Here's the drawing with two shaded views (mm, measured from the low corner). I have some questions. Give positions to 0.01 mm unless a question says otherwise; leave off trailing zeros. Loops run counter-clockwise (first coordinate to the right, second up) from the corner with the lowest first, then second, coordinate; pieces in that order, holes last. Notation, with made-up numbers: (-35.5, 48.25) -> (14.5, 48.25) arc R33 cw to (14.5, 85.25) -> close; hole circle Ø6 at (76.5, 48.5). An arc over 180 degrees is marked (long way). Answer in a Markdown table with one row per item. Add a question column.
Item 1: If we section it at B-B (x = 4): Write out the boundary of the cut face in (y, z), then the cut area to 3 significant figures.
Item 2: If we section it at A-A (z = 12.5): Write out the boundary of the cut face in (x, y).
Item 3: If I drill on line 1 (X direction, y = 25, z = 12.5); line 2 (X direction, y = 43, z = 11.75), over which ranges is the centre line in solid material (lowest first)?
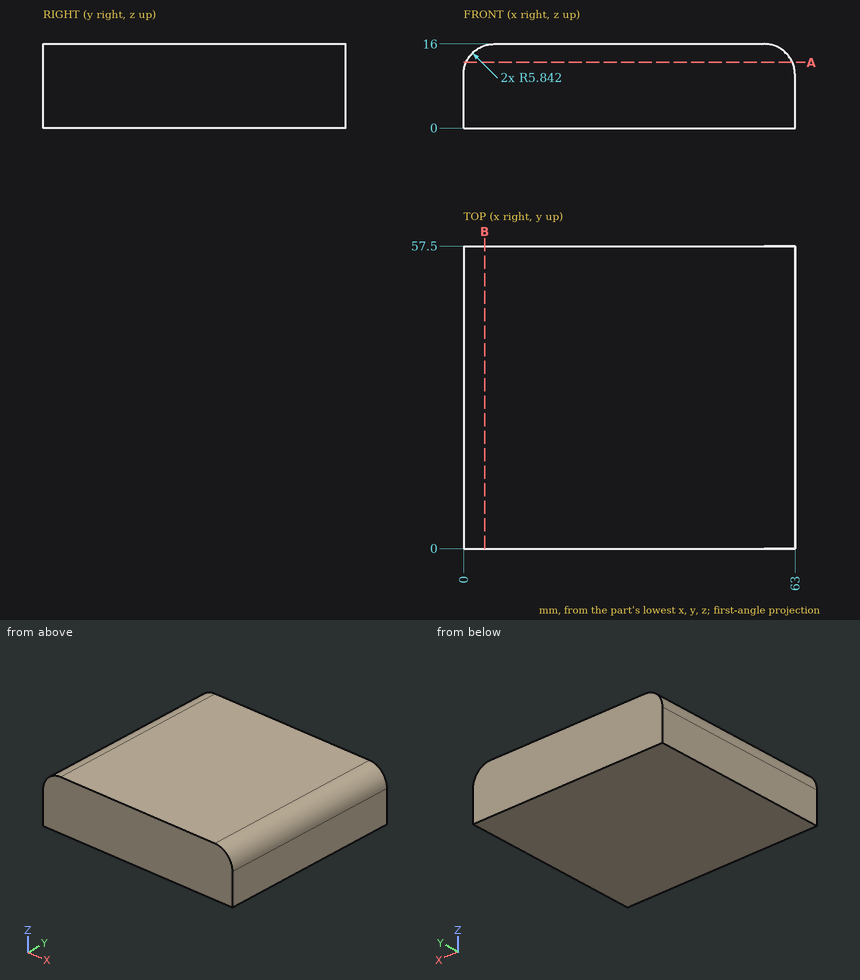
Recorded:
| question | item | result |
|---|---|---|
| 1 | outline | (0, 0) -> (57.5, 0) -> (57.5, 15.7) -> (0, 15.7) -> close |
| 1 | area | 903 mm^2 |
| 2 | outline | (0.49, 0) -> (62.51, 0) -> (62.51, 57.5) -> (0.49, 57.5) -> close |
| 3 | line 1 | x = 0.49 to 62.51 |
| 3 | line 2 | x = 0.22 to 62.78 |
